from build123d import *

# Parameters (mm, degrees)
SKETCH1_W           = 304.8
SKETCH1_H           = 190.5
BOSS_EXTRUDE1_DEPTH = 6.35
SKETCH2_R           = 3.2639
CUT_EXTRUDE1_DEPTH  = 180.829488683
SKETCH3_W           = 25.4
SKETCH3_H           = 50.8
SKETCH3_R           = 3.2639
BOSS_EXTRUDE2_DEPTH = 6.35
FILLET1_R           = 5.08


with BuildPart() as part:
    # Sketch1 → Boss-Extrude1 (new body)
    with BuildSketch(Plane.XY):
        Rectangle(SKETCH1_W, SKETCH1_H)
    extrude(amount=BOSS_EXTRUDE1_DEPTH)

    # Sketch2 → Cut-Extrude1 (cut, through all)
    with BuildSketch(Plane.XY.offset(6.35)):
        with Locations((-114.3, -82.55)):
            Circle(SKETCH2_R)
        with Locations((-88.9, -82.55)):
            Circle(SKETCH2_R)
        with Locations((88.9, -82.55)):
            Circle(SKETCH2_R)
        with Locations((114.3, -82.55)):
            Circle(SKETCH2_R)
    extrude(amount=-CUT_EXTRUDE1_DEPTH, mode=Mode.SUBTRACT)

    # Sketch3 → Boss-Extrude2 (add)
    with BuildSketch(Plane.XY):
        with Locations((-165.1, 69.85)):
            Rectangle(SKETCH3_W, SKETCH3_H)
        with Locations((-165.1, 82.55)):
            Circle(SKETCH3_R, mode=Mode.SUBTRACT)
        with Locations((-165.1, 57.15)):
            Circle(SKETCH3_R, mode=Mode.SUBTRACT)
    boss_extrude2 = extrude(amount=BOSS_EXTRUDE2_DEPTH)

    # Mirror1: Boss-Extrude2 across plane
    add(boss_extrude2.mirror(Plane(origin=(0, 0, 0), x_dir=(0, 0, 1), z_dir=(1, 0, 0))))

    # Fillet1
    fillet1_edges = [part.edges().sort_by_distance(p)[0] for p in [
        (-177.8, 44.45, 3.175),
        (-177.8, 95.25, 3.175),
        (-152.4, 44.45, 3.175),
        (152.4, 44.45, 3.175),
        (177.8, 44.45, 3.175),
        (177.8, 95.25, 3.175),
        (152.4, -95.25, 3.175),
        (-152.4, -95.25, 3.175),
    ]]
    fillet(fillet1_edges, radius=FILLET1_R)


solid = part.part
Read the model definition and answer for the solid it produces. Units are mm, in the model's axes. A direction names the side the tool comes from. Coordinates: 2 decimals unless noted, no trailing zeros. Order: outer loops, then holes, each group sorted by start corner. A loop starts at its lowest first (then second) coordinate and runs counter-clockwise, first axis right, second up. Notation, with made-up numbers: (-19, -3.75) - (-8, -3.75) arc R32 ccw to (-8, 24.25) - close; hole circle Ø11 at (72, -37.5). An arc over 180 degrees is marked (long way). Use one line per item in the form item = value.
(1) Given pin 1 Ø1.9 at (x, z) = (165, 4) entering from -Y, flat-ended and moving along its own axis, determine where the tip first touches the part or whether it passes through.
Computed values:
pin_1 = 44.45
(2) For a pull along Y with two mould halves and no side action, classify faces 1 (the face through (-152.4, -26, 3)), 2 (the face through (85.64, -82.41, 3.22)), 3 (the face through (165, 44.45, 3)), 4 (the face through (2, 95.25, 3)) as pulls with the +Y half, pulls with the -Y half, needs draft (parallel to the pull), parting line crosses it, or undercut.
Computed values:
face_1 = needs draft
face_2 = undercut
face_3 = pulls with the -Y half
face_4 = pulls with the +Y half
(3) Straight lines are drawn through the part: L1, parallel to Y at x = -165.1, z = 1.75; L2, parallel to X at y = 4.5, z = 3.5; L3, parallel to Y at x = -161, z = 2.25. For each, find the intervals that lie inside material, in ascending order.
Computed values:
L1 = 44.45 to 53.89, 60.41 to 79.29, 85.81 to 95.25
L2 = -152.4 to 152.4
L3 = 44.45 to 95.25
(4) Section B-B, the plane z = 3.25 is taken. Give the number of separate pieces and of enclosed holes in the cut face, then the cut area to 3 significant figures.
Computed values:
separate_pieces = 1
enclosed_holes = 8
area = 60,400 mm²
(5) Which of the six approach directions +Z, -Z, +X, -X, +Y, -Y give full straight-line access (tool end or side, diameter ignored) to faces 5 (the face through (152.4, -26, 3)), 6 (the face through (-165, 44.45, 3)), 7 (the face through (-91.306, -80.344, 3.219))?
Computed values:
face_5 = +Z, -Z, +X, -Y
face_6 = +Z, -Z, -X, -Y
face_7 = +Z, -Z
(6) Section D-D, the plane x = -165.1 is taken. Give the vertices of the cut face in (y, z), then the cut area to 3 significant figures.
Computed values:
outline = (44.45, 0) - (53.89, 0) - (53.89, 6.35) - (44.45, 6.35) - close; (60.41, 0) - (79.29, 0) - (79.29, 6.35) - (60.41, 6.35) - close; (85.81, 0) - (95.25, 0) - (95.25, 6.35) - (85.81, 6.35) - close
area = 240 mm²
(7) Section C-C, the plane x = -114.3 is taken. Give the vertices of the cut face in (y, z).
Computed values:
outline = (-95.25, 0) - (-85.81, 0) - (-85.81, 6.35) - (-95.25, 6.35) - close; (-79.29, 0) - (95.25, 0) - (95.25, 6.35) - (-79.29, 6.35) - close
(8) Section A-A, the plane y = -82.55 is taken. Give the vertices of the cut face in (x, z).
Computed values:
outline = (-152.4, 0) - (-117.56, 0) - (-117.56, 6.35) - (-152.4, 6.35) - close; (-111.04, 0) - (-92.16, 0) - (-92.16, 6.35) - (-111.04, 6.35) - close; (-85.64, 0) - (85.64, 0) - (85.64, 6.35) - (-85.64, 6.35) - close; (92.16, 0) - (111.04, 0) - (111.04, 6.35) - (92.16, 6.35) - close; (117.56, 0) - (152.4, 0) - (152.4, 6.35) - (117.56, 6.35) - close
